from build123d import *

# Parameters (mm, degrees)
SKETCH1_W           = 15.875
SKETCH1_H           = 12.7
BOSS_EXTRUDE1_DEPTH = 2.54
FILLET1_R           = 0.635
SHELL1_START        = 0.635
SHELL1_OUTLINE_W    = 1.905
SHELL1_OUTLINE_H    = 11.43
SHELL1_DEPTH        = 14.605
SKETCH2_R           = 2.54
BOSS_EXTRUDE2_DEPTH = 1.905
SKETCH3_W           = 0.569871795
SKETCH3_H           = 3.256410256
BOSS_EXTRUDE3_DEPTH = 0.00254


# Read off the part's stored shape, not the designer's step: Shell1
with BuildPart() as part:
    # Sketch1 → Boss-Extrude1 (new body)
    with BuildSketch(Plane(origin=(0, 0, 0), x_dir=(1, 0, 0), z_dir=(0, 1, 0))):
        with Locations((7.9375, 6.35)):
            Rectangle(SKETCH1_W, SKETCH1_H)
    extrude(amount=BOSS_EXTRUDE1_DEPTH)

    # Fillet1
    fillet1_edges = [part.edges().sort_by_distance(p)[0] for p in [
        (0, 1.27, -12.7),
        (15.875, 1.27, -12.7),
        (15.875, 1.27, 0),
        (0, 1.27, 0),
    ]]
    fillet(fillet1_edges, radius=FILLET1_R)

    # Shell1 outline → Shell1 (cut)
    with BuildSketch(Plane.YZ.offset(SHELL1_START)):
        with Locations((0.9525, -6.35)):
            Rectangle(SHELL1_OUTLINE_W, SHELL1_OUTLINE_H)
    extrude(amount=SHELL1_DEPTH, mode=Mode.SUBTRACT)

    # Sketch2 → Boss-Extrude2 (add)
    with BuildSketch(Plane(origin=(0, 1.905, 0), x_dir=(-1, 0, 0), z_dir=(0, -1, 0))):
        with Locations(Location((-7.9375, 6.35, 0), (0, 0, 270))):
            Circle(SKETCH2_R)
    extrude(amount=BOSS_EXTRUDE2_DEPTH)

    # Sketch3 → Boss-Extrude3 (add)
    with BuildSketch(Plane(origin=(0, 2.54, 0), x_dir=(1, 0, 0), z_dir=(0, 1, 0))):
        with BuildLine():
            Line((7.279705128, 7.450208734), (6.861841546, 7.050789663))
            add(Edge.make_bspline(
                [(6.861841546, 7.050789663), (6.826394953, 7.0874415), (6.757156652, 7.15903402), (6.645587691, 7.253816208), (6.529560035, 7.332804336), (6.411330769, 7.399327635), (6.288773291, 7.449657252), (6.163304701, 7.486333291), (6.034123843, 7.508693286), (5.946699207, 7.511251666), (5.902726963, 7.512538462)],
                knots=[0, 0, 0, 0, 1.115251505, 2.178435587, 3.19620269, 4.182487026, 5.141301733, 6.088180966, 7.038406374, 8, 8, 8, 8], degree=3))
            add(Edge.make_bspline(
                [(5.902726963, 7.512538462), (5.866004796, 7.511521848), (5.793537645, 7.509515672), (5.687136877, 7.494808428), (5.585359044, 7.469798119), (5.487855743, 7.435329281), (5.394913883, 7.390728433), (5.3063386, 7.336030097), (5.222348271, 7.271728275), (5.144052361, 7.198155668), (5.072430014, 7.117772066), (5.00914711, 7.032002955), (4.956137527, 6.941044826), (4.912633425, 6.845818837), (4.87874541, 6.745884235), (4.854545111, 6.6413083), (4.840548304, 6.531966489), (4.838459187, 6.457636741), (4.837397436, 6.419860176)],
                knots=[0, 0, 0, 0, 1.035432265, 2.043311493, 3.022114605, 3.98653278, 4.95457646, 5.923598177, 6.917315552, 7.932509744, 8.948865224, 9.949768934, 10.933144597, 11.912367597, 12.897413939, 13.903909035, 14.934704909, 16, 16, 16, 16], degree=3))
            add(Edge.make_bspline(
                [(4.837397436, 6.419860176), (4.83770342, 6.39334594), (4.838306522, 6.341085836), (4.844908537, 6.263778637), (4.855539337, 6.188772378), (4.870924739, 6.116180674), (4.890164335, 6.045940615), (4.912736762, 5.977446244), (4.941053539, 5.911643999), (4.97248559, 5.847769629), (5.009040702, 5.787566028), (5.048453857, 5.730156898), (5.091190988, 5.675823652), (5.137528908, 5.624788408), (5.188119763, 5.577848731), (5.241655968, 5.533593089), (5.299040605, 5.493129351), (5.359081648, 5.455442035), (5.422297778, 5.422702743), (5.486973793, 5.39304727), (5.554090313, 5.368962616), (5.622830153, 5.349548188), (5.692947662, 5.333039117), (5.765128654, 5.322873974), (5.83874741, 5.315176031), (5.888501332, 5.314700728), (5.913539263, 5.314461538)],
                knots=[0, 0, 0, 0, 1.103660481, 2.175337485, 3.227646561, 4.255952547, 5.262355991, 6.258840057, 7.255597736, 8.242457506, 9.22035537, 10.185017736, 11.140346927, 12.096287581, 13.051739095, 14.01125915, 14.986044842, 15.97314143, 16.960198552, 17.947847494, 18.933482797, 19.925264591, 20.920966487, 21.929612487, 22.958107872, 24, 24, 24, 24], degree=3))
            add(Edge.make_bspline(
                [(5.913539263, 5.314461538), (5.956007897, 5.315689957), (6.039447719, 5.318103479), (6.161907656, 5.336976883), (6.278599775, 5.368022564), (6.37183622, 5.40468571), (6.444884512, 5.440891042), (6.500495097, 5.474379191), (6.558000776, 5.511839363), (6.616446429, 5.554685345), (6.676489454, 5.602402968), (6.737069952, 5.656037337), (6.799738796, 5.713822348), (6.840792535, 5.755064647), (6.861841546, 5.776210337)],
                knots=[0, 0, 0, 0, 1.404581149, 2.759636711, 4.088442092, 5.392261763, 6.066678138, 6.783632037, 7.538459478, 8.336747902, 9.180226004, 10.074962426, 11.012997595, 12, 12, 12, 12], degree=3))
            Line((6.861841546, 5.776210337), (7.266984776, 5.350714543))
            add(Edge.make_bspline(
                [(7.266984776, 5.350714543), (7.238505387, 5.323218588), (7.182919712, 5.269552363), (7.099070264, 5.193351332), (7.015326343, 5.124876235), (6.933711029, 5.061641725), (6.852887378, 5.005489979), (6.77286396, 4.956364915), (6.694546676, 4.91302409), (6.616309243, 4.876198427), (6.537664826, 4.844929614), (6.456748963, 4.818009219), (6.373314287, 4.795235533), (6.286851216, 4.776860159), (6.198166225, 4.76212559), (6.106429341, 4.752179841), (6.012222221, 4.745493645), (5.948320072, 4.744892834), (5.916083333, 4.744589744)],
                knots=[0, 0, 0, 0, 1.244526981, 2.429050516, 3.560637417, 4.644440555, 5.67424972, 6.652764056, 7.595344123, 8.486817594, 9.369275933, 10.254498637, 11.166417451, 12.086725134, 13.032340136, 13.991389299, 14.986715468, 16, 16, 16, 16], degree=3))
            add(Edge.make_bspline(
                [(5.916083333, 4.744589744), (5.856868437, 4.746099249), (5.741001344, 4.749052933), (5.57120114, 4.770937726), (5.409895505, 4.807627196), (5.256692012, 4.859516227), (5.111639375, 4.925802032), (4.974774704, 5.007065316), (4.846318595, 5.103090176), (4.727308719, 5.212751107), (4.619658622, 5.333862399), (4.524508403, 5.463902701), (4.445800139, 5.603511114), (4.380446971, 5.750625175), (4.329341653, 5.905916222), (4.293372173, 6.069552234), (4.271190057, 6.24137521), (4.268763302, 6.358734263), (4.267525641, 6.418588141)],
                knots=[0, 0, 0, 0, 1.078019885, 2.10938526, 3.111377082, 4.085535484, 5.04941344, 6.010039228, 6.978205633, 7.964457913, 8.951525778, 9.924444315, 10.892603023, 11.863865945, 12.85144698, 13.863884204, 14.910567087, 16, 16, 16, 16], degree=3))
            add(Edge.make_bspline(
                [(4.267525641, 6.418588141), (4.268048616, 6.45762433), (4.269085026, 6.534984515), (4.279977786, 6.648942336), (4.295162928, 6.760030827), (4.319252774, 6.867096523), (4.348290707, 6.971581794), (4.384403193, 7.072351009), (4.427532553, 7.169693788), (4.476288628, 7.263773089), (4.531445888, 7.353972592), (4.593062603, 7.43951734), (4.659552517, 7.521067724), (4.732513276, 7.597541827), (4.810884664, 7.669611105), (4.895020519, 7.736885002), (4.984414805, 7.800328301), (5.07930948, 7.858304953), (5.177860994, 7.910747916), (5.278826351, 7.95700485), (5.381957492, 7.995664994), (5.486818369, 8.027732158), (5.593852019, 8.051668028), (5.702294461, 8.06978671), (5.813068412, 8.079915169), (5.887443523, 8.081573262), (5.92498758, 8.082410256)],
                knots=[0, 0, 0, 0, 1.071919942, 2.124283339, 3.142214191, 4.149696895, 5.136002878, 6.119640489, 7.086990633, 8.058538607, 9.028339693, 9.988281803, 10.952401235, 11.916291999, 12.888973767, 13.874849856, 14.873389453, 15.898127285, 16.927174885, 17.938320013, 18.946391617, 19.950418109, 20.947802303, 21.956882652, 22.968648068, 24, 24, 24, 24], degree=3))
            add(Edge.make_bspline(
                [(5.92498758, 8.082410256), (5.95701651, 8.08193047), (6.020741359, 8.080975887), (6.115638353, 8.073018393), (6.209776405, 8.060521229), (6.302818472, 8.041665671), (6.395430086, 8.01928174), (6.486394226, 7.98997307), (6.577145903, 7.957303034), (6.666261809, 7.918252678), (6.753866337, 7.875625686), (6.837907215, 7.827263816), (6.91979548, 7.776143202), (6.997716537, 7.719238304), (7.073130016, 7.658613168), (7.145641572, 7.593984943), (7.214614876, 7.524276087), (7.257898691, 7.475022665), (7.279705128, 7.450208734)],
                knots=[0, 0, 0, 0, 0.996412454, 1.982464992, 2.961075852, 3.949442424, 4.934965278, 5.923860011, 6.921385422, 7.934793307, 8.949617135, 9.951082467, 10.950285876, 11.951772932, 12.951063433, 13.960125323, 14.972308753, 16, 16, 16, 16], degree=3))
        make_face()
        Polygon((7.808871795, 8.082410256), (8.37874359, 8.082410256), (8.37874359, 7.146192308), (8.745089744, 7.146192308), (8.745089744, 6.657730769), (8.37874359, 6.657730769), (8.37874359, 4.826), (7.808871795, 4.826), (7.808871795, 6.657730769), (7.523935897, 6.657730769), (7.523935897, 7.146192308), (7.808871795, 7.146192308), align=None)
        with BuildLine():
            Line((8.989320513, 7.146192308), (9.477782051, 7.146192308))
            Line((9.477782051, 7.146192308), (9.477782051, 6.860620393))
            add(Edge.make_bspline(
                [(9.477782051, 6.860620393), (9.49159969, 6.885999247), (9.51860684, 6.935603272), (9.568221237, 7.002186851), (9.625220267, 7.058261684), (9.687555778, 7.105000626), (9.755416695, 7.141429043), (9.826985825, 7.167388882), (9.901650896, 7.18425918), (9.952584876, 7.186011685), (9.978327925, 7.186897436)],
                knots=[0, 0, 0, 0, 1.09866127, 2.147379032, 3.14564304, 4.131443017, 5.102343063, 6.064490016, 7.021754664, 8, 8, 8, 8], degree=3))
            add(Edge.make_bspline(
                [(9.978327925, 7.186897436), (9.99702059, 7.186022129), (10.035085533, 7.184239691), (10.093101861, 7.173878355), (10.151955263, 7.155143087), (10.190685873, 7.138274469), (10.210474359, 7.129655849)],
                knots=[0, 0, 0, 0, 0.931404136, 1.896671404, 2.925354185, 4, 4, 4, 4], degree=3))
            Line((10.210474359, 7.129655849), (10.033661458, 6.64691847))
            add(Edge.make_bspline(
                [(10.033661458, 6.64691847), (10.01785691, 6.654554463), (9.988150443, 6.668907192), (9.945021811, 6.68584489), (9.905880789, 6.696179446), (9.8810661, 6.697721452), (9.86956891, 6.698435897)],
                knots=[0, 0, 0, 0, 1.214386998, 2.282580073, 3.20428172, 4, 4, 4, 4], degree=3))
            add(Edge.make_bspline(
                [(9.86956891, 6.698435897), (9.858713328, 6.697962468), (9.837358527, 6.697031151), (9.805839437, 6.689050083), (9.776155019, 6.675286977), (9.746874781, 6.657655073), (9.720308609, 6.633145407), (9.693758846, 6.604771118), (9.670361774, 6.569739283), (9.645671077, 6.530747072), (9.624647831, 6.483020641), (9.606621046, 6.426045117), (9.590559035, 6.359161255), (9.579506178, 6.282013934), (9.568823149, 6.195349687), (9.562464348, 6.098532411), (9.557725052, 5.991868249), (9.557435276, 5.917412815), (9.557284255, 5.878609175)],
                knots=[0, 0, 0, 0, 0.544232178, 1.070598461, 1.618251235, 2.182094276, 2.777567932, 3.425210017, 4.127676488, 4.886675562, 5.738955394, 6.734782583, 7.883056018, 9.186093582, 10.642914445, 12.264202625, 14.053029461, 16, 16, 16, 16], degree=3))
            Line((9.557284255, 5.878609175), (9.559192308, 5.765398037))
            Line((9.559192308, 5.765398037), (9.559192308, 4.826))
            Line((9.559192308, 4.826), (8.989320513, 4.826))
            Line((8.989320513, 4.826), (8.989320513, 7.146192308))
        make_face()
        with Locations((10.739641026, 6.454205128)):
            Rectangle(SKETCH3_W, SKETCH3_H)
    extrude(amount=BOSS_EXTRUDE3_DEPTH)


solid = part.part
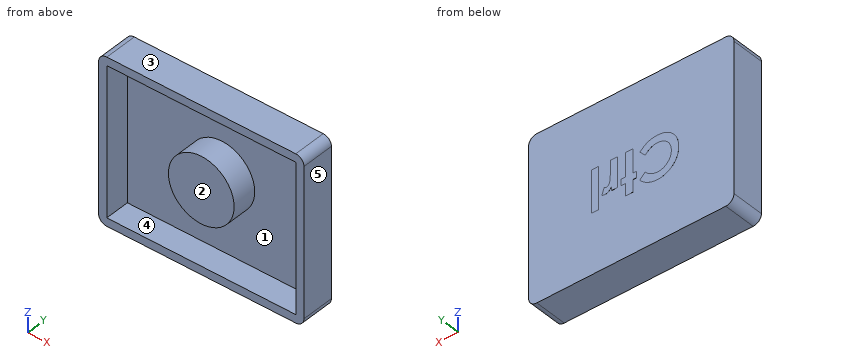
Can you work these out from the model? Positions are in its coordinate system, mm. Face numbers are marked on the shaded views. A direction names the side the tool comes from. Round coordinates to 2 decimals unless told otherwise and drop trailing zeros. Order: outer loops, then holes, each group sorted by start corner. A loop starts at its lowest first (then second) coordinate and runs counter-clockwise, first axis right, second up. Notation, with made-up numbers: M 7.25,31 L 64.25,31 A24 ccw 64.25,44 Z; hole C 84.5,-27.5 d6. An arc over 180 degrees is marked long. Use a Markdown table: item, result.
1) On a 3-axis mill with a long thin cutter (end or side, diameter ignored), from which of +Z, -Z, +X, -X, +Y, -Y can I reach the whole of each face in a straight line? I mean the marked faces 1 and 2. Say none if no direction works.
Geometry says:
| item | result |
|---|---|
| face 1 | -Y |
| face 2 | +Z, -Z, +X, -X, -Y |
2) If we mould it in two halves opening along Z, with no side actions, what happens to the marked faces 3, 4 and 5? For each: +Z half, -Z half, draft (parallel to the pull), parting line (faces both ways), or undercut.
Geometry says:
| item | result |
|---|---|
| face 3 | +Z half |
| face 4 | undercut |
| face 5 | draft |
3) If I drill on line 1 along Z through (x, y) = (13.5, 1.35) (3 decimals); line 2 along X through (y, z) = (0.1, -5.25) (3 decimals); line 3 along Z through (x, y) = (9.75, 1.15) (3 decimals), over which ranges is the centre line in solid material (lowest first)?
Geometry says:
| item | result |
|---|---|
| line 1 | z = -12.7 to -12.065, -0.635 to 0 |
| line 2 | x = 0 to 0.635, 5.648 to 10.227, 15.24 to 15.875 |
| line 3 | z = -12.7 to -12.065, -8.129 to -4.571, -0.635 to 0 |
4) Imagine slicing it at B-B (x = 3.5). List the corners of the cut face in (y, z) for me (3 decimals).
Geometry says:
| item | result |
|---|---|
| outline | M 0,-12.7 L 2.54,-12.7 L 2.54,0 L 0,0 L 0,-0.635 L 1.905,-0.635 L 1.905,-12.065 L 0,-12.065 Z |
5) Imagine slicing it at C-C (z = -4.25). List the corners of the cut face in (x, y) for me (3 decimals), then the cut area to 3 significant figures.
Geometry says:
| item | result |
|---|---|
| outline | M 0,0 L 0.635,0 L 0.635,1.905 L 6.509,1.905 L 6.509,0 L 9.366,0 L 9.366,1.905 L 15.24,1.905 L 15.24,0 L 15.875,0 L 15.875,2.54 L 0,2.54 Z |
| area | 17.9 mm² |
6) Imagine slicing it at D-D (z = -2.75). List the corners of the cut face in (x, y) for me (3 decimals), then the cut area to 3 significant figures.
Geometry says:
| item | result |
|---|---|
| outline | M 0,0 L 0.635,0 L 0.635,1.905 L 15.24,1.905 L 15.24,0 L 15.875,0 L 15.875,2.54 L 0,2.54 Z |
| area | 12.5 mm² |
7) I'm going to push a flat-ended pin straight in: P1, Ø3.5, axis at x = 11, z = -6.5, coming from the -Y side. Where does the tip first touch, or does it pass through?
Geometry says:
| item | result |
|---|---|
| P1 | stops at y = 0 |
8) Imagine slicing it at A-A (y = 0.9). Give the number of separate pieces and of enclosed holes in the cut face, then the cut area to 3 significant figures.
Geometry says:
| item | result |
|---|---|
| separate pieces | 2 |
| enclosed holes | 1 |
| area | 54.6 mm² |
